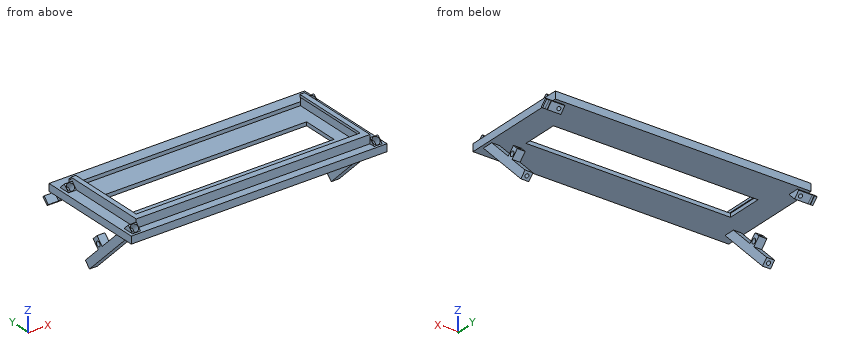
from build123d import *

# Parameters (mm, degrees)
SKETCH2_W                       = 210
SKETCH2_H                       = 90
BOSS_EXTRUDE1_DEPTH             = 6
SKETCH3_W                       = 188
SKETCH3_H                       = 70
CUT_EXTRUDE1_DEPTH              = 3
CUT_EXTRUDE2_REACH              = 116.276
SKETCH4_W                       = 168
SKETCH4_H                       = 30
BOSS_EXTRUDE2_DEPTH             = 9
CUT_EXTRUDE3_DEPTH              = 2.5
SKETCH9_R                       = 3
CUT_EXTRUDE5_DEPTH              = 7
CUT_EXTRUDE7_DEPTH              = 2.5
CUT_EXTRUDE9_REACH              = 125.918
SKETCH14_R                      = 1.5
SKETCH15_R                      = 3
CUT_EXTRUDE10_DEPTH             = 7
CUT_EXTRUDE12_REACH             = 139.325
SKETCH17_R                      = 1.5
BOSS_EXTRUDE3_DEPTH             = 9
SKETCH19_R                      = 3
CUT_EXTRUDE13_DEPTH             = 7
SKETCH20_R                      = 3
CUT_EXTRUDE14_DEPTH             = 7
CUT_EXTRUDE15_DEPTH             = 2.5
CUT_EXTRUDE16_REACH             = 125.918
SKETCH22_R                      = 1.5
CUT_EXTRUDE16_DIRECTION_2_DEPTH = 124.918371619
CUT_EXTRUDE17_REACH             = 139.325
SKETCH23_R                      = 1.5
CUT_EXTRUDE18_DEPTH             = 2.5
SKETCH25_W                      = 6.5
SKETCH25_H                      = 6
BOSS_EXTRUDE4_DEPTH             = 8
SKETCH26_R                      = 1.4
CUT_EXTRUDE19_DEPTH             = 4
SKETCH27_R                      = 2
CUT_EXTRUDE20_DEPTH             = 217.245809208
BOSS_EXTRUDE6_DEPTH             = 8.5
CUT_EXTRUDE21_REACH             = 145.328
SKETCH29_W                      = 2
SKETCH29_H                      = 0.5
BOSS_EXTRUDE7_DEPTH             = 8.5
CUT_EXTRUDE22_REACH             = 145.328
SKETCH31_W                      = 2
SKETCH31_H                      = 0.5
BOSS_EXTRUDE8_DEPTH             = 5
BOSS_EXTRUDE9_DEPTH             = 2


with BuildPart() as part:
    # Sketch2 → Boss-Extrude1 (new body)
    with BuildSketch(Plane.XY):
        Rectangle(SKETCH2_W, SKETCH2_H)
    extrude(amount=BOSS_EXTRUDE1_DEPTH)

    # Sketch3 → Cut-Extrude1 (cut)
    with BuildSketch(Plane.XY.offset(6)):
        Rectangle(SKETCH3_W, SKETCH3_H)
    extrude(amount=-CUT_EXTRUDE1_DEPTH, mode=Mode.SUBTRACT)

    # Sketch4 → Cut-Extrude2 (cut, up to next)
    with BuildSketch(Plane.XY.offset(3), mode=Mode.PRIVATE) as cut_extrude2_sk1:
        Rectangle(SKETCH4_W, SKETCH4_H)
    cut_extrude2_tool1 = extrude(cut_extrude2_sk1.sketch, amount=-CUT_EXTRUDE2_REACH, mode=Mode.PRIVATE) & part.part
    add(cut_extrude2_tool1.solids().sort_by_distance((0, 0, 3))[0], mode=Mode.SUBTRACT)

    # Sketch7 → Boss-Extrude2 (add)
    with BuildSketch(Plane.ZY.offset(105)):
        Polygon((-6.01040764, 38.98959236), (-1.414213562, 43.585786438), (10.596194078, 31.575378798), (6, 26.97918472), align=None)
        Polygon((-41, 4), (6, -43), (10.596194078, -38.403805922), (-36.403805922, 8.596194078), align=None)
    extrude(amount=-BOSS_EXTRUDE2_DEPTH)

    # Sketch8 → Cut-Extrude3 (cut)
    with BuildSketch(Plane.ZY.offset(105)):
        Polygon((6, 36.171572875), (10.596194078, 31.575378798), (6, 26.97918472), align=None)
        Polygon((6, -33.807611845), (6, -43), (10.596194078, -38.403805922), align=None)
    extrude(amount=-CUT_EXTRUDE3_DEPTH, mode=Mode.SUBTRACT)

    # Sketch9 → Cut-Extrude5 (cut)
    with BuildSketch(Plane(origin=(0, 10.48959236, -10.48959236), x_dir=(1, 0, 0), z_dir=(0, -0.7071067811865437, 0.7071067811865515))):
        with Locations(Location((-99.25, 26.569805153, 0), (0, 0, 270))):
            Circle(SKETCH9_R)
    extrude(amount=-CUT_EXTRUDE5_DEPTH, mode=Mode.SUBTRACT)

    # Sketch11 → Cut-Extrude7 (cut)
    with BuildSketch(Plane.ZY.offset(105)):
        Polygon((-1.414213562, 43.585786438), (0, 42.171572875), (0, 32.97918472), (-6.01040764, 38.98959236), align=None)
        Polygon((-36.403805922, 8.596194078), (-41, 4), (0, -37), (0, -27.807611845), align=None)
    extrude(amount=-CUT_EXTRUDE7_DEPTH, mode=Mode.SUBTRACT)

    # Sketch14 → Cut-Extrude9 (cut, up to next)
    with BuildSketch(Plane(origin=(0, 15.439339828, -15.439339828), x_dir=(1, 0, 0), z_dir=(0, -0.7071067811865437, 0.7071067811865515)), mode=Mode.PRIVATE) as cut_extrude9_sk1:
        with Locations(Location((-99.25, 26.569805153, 0), (0, 0, 270))):
            Circle(SKETCH14_R)
    cut_extrude9_tool1 = extrude(cut_extrude9_sk1.sketch, amount=-CUT_EXTRUDE9_REACH, mode=Mode.PRIVATE) & part.part
    add(cut_extrude9_tool1.solids().sort_by_distance((-99.25, 34.227029, 3.34835))[0], mode=Mode.SUBTRACT)

    # Sketch15 → Cut-Extrude10 (cut)
    with BuildSketch(Plane(origin=(0, -24.5, 24.5), x_dir=(1, 0, 0), z_dir=(0, -0.707106781186551, 0.7071067811865441))):
        with Locations(Location((-99.25, -22.912950904, 0), (0, 0, 270))):
            Circle(SKETCH15_R)
    extrude(amount=-CUT_EXTRUDE10_DEPTH, mode=Mode.SUBTRACT)

    # Sketch17 → Cut-Extrude12 (cut, up to next)
    with BuildSketch(Plane(origin=(0, -19.550252532, 19.550252532), x_dir=(1, 0, 0), z_dir=(0, -0.7071067811865509, 0.7071067811865442)), mode=Mode.PRIVATE) as cut_extrude12_sk1:
        with Locations(Location((-99.25, -22.912950904, 0), (0, 0, 270))):
            Circle(SKETCH17_R)
    cut_extrude12_tool1 = extrude(cut_extrude12_sk1.sketch, amount=-CUT_EXTRUDE12_REACH, mode=Mode.PRIVATE) & part.part
    add(cut_extrude12_tool1.solids().sort_by_distance((-99.25, -35.752155, 3.34835))[0], mode=Mode.SUBTRACT)

    # Sketch18 → Boss-Extrude3 (add)
    with BuildSketch(Plane(origin=(105, 0, 0), x_dir=(0, 0, -1), z_dir=(1, 0, 0))):
        Polygon((-10.596194078, 31.575378798), (1.414213562, 43.585786438), (6.01040764, 38.98959236), (-6, 26.97918472), align=None)
        Polygon((-10.596194078, -38.403805922), (36.403805922, 8.596194078), (41, 4), (-6, -43), align=None)
    extrude(amount=-BOSS_EXTRUDE3_DEPTH)

    # Sketch19 → Cut-Extrude13 (cut)
    with BuildSketch(Plane(origin=(0, 10.48959236, -10.48959236), x_dir=(1, 0, 0), z_dir=(0, -0.7071067811865444, 0.7071067811865508))):
        with Locations(Location((99.25, 26.569805153, 0), (0, 0, 270))):
            Circle(SKETCH19_R)
    extrude(amount=-CUT_EXTRUDE13_DEPTH, mode=Mode.SUBTRACT)

    # Sketch20 → Cut-Extrude14 (cut)
    with BuildSketch(Plane(origin=(0, -24.5, 24.5), x_dir=(1, 0, 0), z_dir=(0, -0.707106781186551, 0.7071067811865441))):
        with Locations(Location((99.25, -22.912950904, 0), (0, 0, 270))):
            Circle(SKETCH20_R)
    extrude(amount=-CUT_EXTRUDE14_DEPTH, mode=Mode.SUBTRACT)

    # Sketch21 → Cut-Extrude15 (cut)
    with BuildSketch(Plane(origin=(105, 0, 0), x_dir=(0, 0, -1), z_dir=(1, 0, 0))):
        Polygon((-10.596194078, -38.403805922), (-6, -33.807611845), (-6, -43), align=None)
        Polygon((-6, 36.171572875), (-6, 26.97918472), (-10.596194078, 31.575378798), align=None)
    extrude(amount=-CUT_EXTRUDE15_DEPTH, mode=Mode.SUBTRACT)

    # Sketch22 → Cut-Extrude16 (cut, up to next)
    with BuildSketch(Plane(origin=(0, 15.439339828, -15.439339828), x_dir=(1, 0, 0), z_dir=(0, -0.7071067811865445, 0.7071067811865507)), mode=Mode.PRIVATE) as cut_extrude16_sk1:
        with Locations(Location((99.25, 26.569805153, 0), (0, 0, 90))):
            Circle(SKETCH22_R)
    cut_extrude16_tool1 = extrude(cut_extrude16_sk1.sketch, amount=-CUT_EXTRUDE16_REACH, mode=Mode.PRIVATE) & part.part
    add(cut_extrude16_tool1.solids().sort_by_distance((99.25, 34.227029, 3.34835))[0], mode=Mode.SUBTRACT)

    # Sketch22 → Cut-Extrude16 direction 2 (cut)
    with BuildSketch(Plane(origin=(0, 15.439339828, -15.439339828), x_dir=(1, 0, 0), z_dir=(0, -0.7071067811865445, 0.7071067811865507))):
        with Locations(Location((99.25, 26.569805153, 0), (0, 0, 90))):
            Circle(SKETCH22_R)
    extrude(amount=CUT_EXTRUDE16_DIRECTION_2_DEPTH, mode=Mode.SUBTRACT)

    # Sketch23 → Cut-Extrude17 (cut, up to next)
    with BuildSketch(Plane(origin=(0, -19.550252532, 19.550252532), x_dir=(1, 0, 0), z_dir=(0, -0.7071067811865509, 0.7071067811865442)), mode=Mode.PRIVATE) as cut_extrude17_sk1:
        with Locations(Location((99.25, -22.912950904, 0), (0, 0, 270))):
            Circle(SKETCH23_R)
    cut_extrude17_tool1 = extrude(cut_extrude17_sk1.sketch, amount=-CUT_EXTRUDE17_REACH, mode=Mode.PRIVATE) & part.part
    add(cut_extrude17_tool1.solids().sort_by_distance((99.25, -35.752155, 3.34835))[0], mode=Mode.SUBTRACT)

    # Sketch24 → Cut-Extrude18 (cut)
    with BuildSketch(Plane(origin=(105, 0, 0), x_dir=(0, 0, -1), z_dir=(1, 0, 0))):
        Polygon((1.414213562, 43.585786438), (0, 42.171572875), (0, 32.97918472), (6.01040764, 38.98959236), align=None)
        Polygon((0, -27.807611845), (0, -37), (41, 4), (36.403805922, 8.596194078), align=None)
    extrude(amount=-CUT_EXTRUDE18_DEPTH, mode=Mode.SUBTRACT)

    # Sketch25 → Boss-Extrude4 (add)
    with BuildSketch(Plane(origin=(0, -13.903805922, -13.903805922), x_dir=(1, 0, 0), z_dir=(0, 0.7071067811865439, 0.7071067811865511))):
        with Locations((-99.25, 8.819805153)):
            Rectangle(SKETCH25_W, SKETCH25_H)
        with Locations((99.25, 8.819805153)):
            Rectangle(SKETCH25_W, SKETCH25_H)
    extrude(amount=BOSS_EXTRUDE4_DEPTH)

    # Sketch26 → Cut-Extrude19 (cut)
    with BuildSketch(Plane(origin=(0, -8.246951673, -8.246951673), x_dir=(1, 0, 0), z_dir=(0, 0.7071067811865438, 0.7071067811865512))):
        with Locations(Location((99.25, 8.819805153, 0), (0, 0, 270))):
            Circle(SKETCH26_R)
        with Locations(Location((-99.25, 8.819805153, 0), (0, 0, 270))):
            Circle(SKETCH26_R)
    extrude(amount=-CUT_EXTRUDE19_DEPTH, mode=Mode.SUBTRACT)

    # Sketch27 → Cut-Extrude20 (cut, through all)
    with BuildSketch(Plane.ZY.offset(102.5)):
        with Locations((-18.019029611, -5.545941546)):
            Circle(SKETCH27_R)
    extrude(amount=-CUT_EXTRUDE20_DEPTH, mode=Mode.SUBTRACT)

    # Sketch28 → Boss-Extrude6 (add)
    with BuildSketch(Plane(origin=(102.5, 0, 0), x_dir=(0, 0, -1), z_dir=(1, 0, 0))):
        Polygon((1.414213562, 43.585786438), (6.01040764, 38.98959236), (4.772970773, 37.752155493), (0.176776695, 42.348349571), align=None)
    extrude(amount=BOSS_EXTRUDE6_DEPTH)

    # Sketch29 → Cut-Extrude21 (cut, up to next)
    with BuildSketch(Plane(origin=(0, 21.085786438, 21.085786438), x_dir=(1, 0, 0), z_dir=(0, 0.7071067811865506, 0.7071067811865446)), mode=Mode.PRIVATE) as cut_extrude21_sk1:
        with Locations((108, 31.569805153)):
            Rectangle(SKETCH29_W, SKETCH29_H)
    cut_extrude21_tool1 = extrude(cut_extrude21_sk1.sketch, amount=-CUT_EXTRUDE21_REACH, mode=Mode.PRIVATE) & part.part
    add(cut_extrude21_tool1.solids().sort_by_distance((108, 43.40901, -1.237437))[0], mode=Mode.SUBTRACT)

    # Sketch30 → Boss-Extrude7 (add)
    with BuildSketch(Plane.ZY.offset(102.5)):
        Polygon((-1.414213562, 43.585786438), (-6.01040764, 38.98959236), (-4.772970773, 37.752155493), (-0.176776695, 42.348349571), align=None)
    extrude(amount=BOSS_EXTRUDE7_DEPTH)

    # Sketch31 → Cut-Extrude22 (cut, up to next)
    with BuildSketch(Plane(origin=(0, 21.085786438, 21.085786438), x_dir=(1, 0, 0), z_dir=(0, 0.7071067811865506, 0.7071067811865446)), mode=Mode.PRIVATE) as cut_extrude22_sk1:
        with Locations((-108, 31.569805153)):
            Rectangle(SKETCH31_W, SKETCH31_H)
    cut_extrude22_tool1 = extrude(cut_extrude22_sk1.sketch, amount=-CUT_EXTRUDE22_REACH, mode=Mode.PRIVATE) & part.part
    add(cut_extrude22_tool1.solids().sort_by_distance((-108, 43.40901, -1.237437))[0], mode=Mode.SUBTRACT)

    # Sketch32 → Boss-Extrude8 (add)
    with BuildSketch(Plane.XY.offset(6)):
        Polygon((-96, -38.403805922), (96, -38.403805922), (96, 35), (94, 35), (94, -35), (-94, -35), (-94, 35), (-96, 35), align=None)
    extrude(amount=BOSS_EXTRUDE8_DEPTH)

    # Sketch33 → Boss-Extrude9 (add)
    with BuildSketch(Plane.XY.offset(11)):
        Polygon((-96, -38.403805922), (96, -38.403805922), (96, 33), (92, 33), (92, -33), (-92, -33), (-92, 33), (-96, 33), align=None)
    extrude(amount=BOSS_EXTRUDE9_DEPTH)


solid = part.part
Here's how the part is built. I have some questions about the finished solid (model axes, mm). Coordinates: 2 decimals unless noted, no trailing zeros. Loops run counter-clockwise (first coordinate to the right, second up) from the corner with the lowest first, then second, coordinate; pieces in that order, holes last. Notation, with made-up numbers: (-14.75, 33.5) -> (-7.75, 33.5) arc R32 cw to (-7.75, 67.5) -> close; hole circle Ø5 at (5.5, 45). An arc over 180 degrees is marked (long way). Use one line per item in the form item = value. Start each with the question number.
(1) If we section it at A-A (x = 43): Please give me the cut outline in (y, z), then the cut area to 3 significant figures.
(2) If we section it at B-B (y = 21): Please give me the cut outline in (x, z), then the cut area to 3 significant figures.
(3) Will these pins go through, and if not, where does the flat tip stop? pin 1 (0.6 mm diameter, centred on y = -7.5, z = 11.5, fed in from -X); pin 2 (10 mm diameter, centred on y = -15, z = -34.5, fed in from +X); pin 3 (12 mm diameter, centred on x = 1.5, y = 17, fed in from -Z); pin 4 (0.6 mm diameter, centred on x = 94, z = 12, fed in from +Y).
(4) If we section it at C-C (z = -30): Give the number of separate pieces and of enclosed holes in the cut face, then the cut area to 3 significant figures.
(5) Please list where these lines run through material, in increasing order: line 1 along X through (y, z) = (-33.5, 2.5); line 2 along Z through (x, y) = (-93, -10.5); line 3 along Y through (x, z) = (-41.5, 4).
Verdict:
q1.outline = (-45, 0) -> (-15, 0) -> (-15, 3) -> (-35, 3) -> (-35, 11) -> (-33, 11) -> (-33, 13) -> (-38.4, 13) -> (-38.4, 6) -> (-45, 6) -> close; (15, 0) -> (45, 0) -> (45, 6) -> (35, 6) -> (35, 3) -> (15, 3) -> close
q1.area = 268 mm²
q2.outline = (-105, 0) -> (105, 0) -> (105, 6) -> (96, 6) -> (96, 13) -> (92, 13) -> (92, 11) -> (94, 11) -> (94, 3) -> (-94, 3) -> (-94, 11) -> (-92, 11) -> (-92, 13) -> (-96, 13) -> (-96, 6) -> (-105, 6) -> close
q2.area = 732 mm²
q3.pin_1 = -96
q3.pin_2 = through
q3.pin_3 = 0
q3.pin_4 = 33
q4.separate_pieces = 2
q4.enclosed_holes = 2
q4.area = 99.5 mm²
q5.line_1 = -105 to -100.37, -98.13 to 98.13, 100.37 to 105
q5.line_2 = 0 to 3, 11 to 13
q5.line_3 = -45 to -35, 35 to 45
